Geometry: final body of the model. Coordinates: model frame, mm. A direction names the side the tool comes from. Round coordinates to 2 decimals unless told otherwise and drop trailing zeros. Loops run counter-clockwise (first coordinate to the right, second up) from the corner with the lowest first, then second, coordinate; pieces in that order, holes last. Notation, with made-up numbers: (43, 11.5) - (49, 11.5) arc R21 ccw to (49, 31.5) - close; hole circle Ø7 at (65, 3). An arc over 180 degrees is marked (long way). Answer as CSV lines item,"result".
Autodesk Inventor part; units mm, degrees
ref_plane "YZ Plane" through (0, 0, 0) normal (1, 0, 0) x (0, 1, 0)
ref_plane "XZ Plane" through (0, 0, 0) normal (0, 1, 0) x (-1, 0, 0)
ref_plane "XY Plane" through (0, 0, 0) normal (0, 0, 1) x (1, 0, 0)
sketch "Sketch1" plane through (0, 0, 0) normal (0, 0, 1) x (1, 0, 0)
  circle A0 centre (0, 0) radius 25.4
  dimension "d0" = 50.8
extrude "Extrusion1" add sketch "Sketch1" along normal blind 11.43
sketch "Sketch2" plane through (0, 0, 11.43) normal (0, 0, 1) x (1, 0, 0)
  line L0 (0, 0) -> (-6.35, 0)
  line L1 (0, 0) -> (6.35, 0)
  line L2 (-6.35, 0) -> (-6.35, 6.35)
  line L3 (-6.35, 6.35) -> (-12.7, 6.35)
  line L4 (-12.7, 6.35) -> (-12.7, -6.35)
  line L5 (-12.7, -6.35) -> (-6.35, -6.35)
  line L6 (-6.35, -6.35) -> (-6.35, 0)
  line L7 (6.35, 0) -> (6.35, 6.35)
  line L8 (6.35, 6.35) -> (12.7, 6.35)
  line L9 (12.7, 6.35) -> (12.7, -6.35)
  line L10 (12.7, -6.35) -> (6.35, -6.35)
  line L11 (6.35, -6.35) -> (6.35, 0)
  dimension "d3" = 6.35
  dimension "d4" = 6.35
  dimension "d5" = 6.35
  dimension "d6" = 6.35
  dimension "d7" = 12.7
  dimension "d8" = 6.35
  dimension "d9" = 6.35
  dimension "d10" = 12.7
extrude "Extrusion2" add sketch "Sketch2" along normal blind 22.86
sketch "Sketch3" plane through (0, 0, 34.29) normal (0, 0, 1) x (1, 0, 0)
  line L0 (-12.7, 6.35) -> (-12.7, -6.35)
  line L1 (-12.7, -6.35) -> (-12.7, -8.89)
  line L2 (-12.7, -8.89) -> (-15.24, -8.89)
  line L3 (-15.24, -8.89) -> (15.24, -8.89)
  line L4 (15.24, -8.89) -> (15.24, 8.89)
  line L5 (15.24, 8.89) -> (-15.24, 8.89)
  line L6 (-15.24, 8.89) -> (-15.24, -8.89)
  point P0 (0, 0)
  dimension "d13" = 2.54
  dimension "d14" = 2.54
  dimension "d15" = 30.48
  dimension "d16" = 17.78
extrude "Extrusion3" add sketch "Sketch3" along normal blind 25.4
sketch "Sketch4" plane through (-15.24, -8.89, 34.29) normal (-1, 0, 0) x (0, 0, 1)
  line L0 (0, 17.78) -> (25.4, 17.78)
  line L1 (0, 17.78) -> (0, 12.7)
  line L2 (0, 0) -> (0, 17.78)
  line L3 (0, 12.7) -> (15.24, 12.7)
  line L4 (15.24, 12.7) -> (15.24, 5.08)
  line L5 (15.24, 5.08) -> (21.59, 5.08)
  line L6 (21.59, 5.08) -> (21.59, 12.7)
  line L7 (21.59, 12.7) -> (15.24, 12.7)
  point P0 (-34.29, 8.89)
  dimension "d19" = 5.08
  dimension "d20" = 15.24
  dimension "d21" = 7.62
  dimension "d22" = 6.35
  dimension "d23" = 7.62
extrude "Extrusion4" add sketch "Sketch4" along normal blind 10.16
sketch "Sketch5" plane through (15.24, -8.89, 34.29) normal (1, 0, 0) x (0, 0, -1)
  line L0 (0, 0) -> (0, 5.08)
  line L1 (0, 17.78) -> (0, 0)
  line L2 (0, 5.08) -> (-15.24, 5.08)
  line L3 (-15.24, 5.08) -> (-21.59, 5.08)
  line L4 (-21.59, 5.08) -> (-21.59, 12.7)
  line L5 (-21.59, 12.7) -> (-15.24, 12.7)
  line L6 (-15.24, 12.7) -> (-15.24, 5.08)
  point P0 (34.29, 8.89)
  dimension "d26" = 5.08
  dimension "d27" = 15.24
  dimension "d28" = 6.35
  dimension "d29" = 7.62
extrude "Extrusion5" add sketch "Sketch5" along normal blind 10.16
sketch "Sketch6" plane through (0, 0, 59.69) normal (0, 0, 1) x (1, 0, 0)
  line L0 (-15.24, -8.89) -> (15.24, -8.89)
  line L1 (15.24, -8.89) -> (4.445, -8.89)
  line L2 (-15.24, 8.89) -> (-15.24, -8.89)
  line L3 (-15.24, -8.89) -> (-4.445, -8.89)
  line L4 (-4.445, -8.89) -> (-4.445, -3.81)
  line L5 (15.24, 8.89) -> (-15.24, 8.89)
  line L6 (-4.445, -3.81) -> (4.445, -3.81)
  line L7 (4.445, -3.81) -> (4.445, 3.81)
  line L8 (4.445, 3.81) -> (-4.445, 3.81)
  line L9 (-4.445, 3.81) -> (-4.445, -3.81)
  point P0 (0, 0)
  dimension "d32" = 10.795
  dimension "d33" = 10.795
  dimension "d34" = 5.08
  dimension "d35" = 7.62
extrude "Extrusion6" add sketch "Sketch6" along normal blind 6.35
sketch "Sketch7" plane through (0, 0, 66.04) normal (0, 0, 1) x (1, 0, 0)
  line L0 (4.445, 3.81) -> (4.445, -3.81)
  line L1 (4.445, 3.81) -> (8.255, 3.81)
  line L2 (8.255, 3.81) -> (8.255, 6.35)
  line L3 (12.7, 6.35) -> (6.35, 6.35)
  line L4 (-12.7, -6.35) -> (-6.35, -6.35)
  line L5 (8.255, 6.35) -> (-8.255, 6.35)
  line L6 (-8.255, 6.35) -> (-8.255, -6.35)
  line L7 (-8.255, -6.35) -> (8.255, -6.35)
  line L8 (8.255, -6.35) -> (8.255, 6.35)
  point P0 (0, 0)
  dimension "d38" = 3.81
  dimension "d39" = 16.51
extrude "Extrusion7" add sketch "Sketch7" along normal blind 15.24
sketch "Sketch8" plane through (0, 0, 81.28) normal (0, 0, 1) x (1, 0, 0)
  line L0 (-8.255, 6.35) -> (-8.255, -6.35)
  line L1 (-8.255, -6.35) -> (-8.255, -7.62)
  line L2 (-8.255, -7.62) -> (-9.525, -7.62)
  line L3 (-9.525, -7.62) -> (9.525, -7.62)
  line L4 (9.525, -7.62) -> (9.525, 7.62)
  line L5 (9.525, 7.62) -> (-9.525, 7.62)
  line L6 (-9.525, 7.62) -> (-9.525, -7.62)
  point P0 (0, 0)
  dimension "d42" = 1.27
  dimension "d43" = 1.27
  dimension "d44" = 15.24
extrude "Extrusion8" add sketch "Sketch8" along normal blind 12.7
sketch "Sketch9" plane through (-9.525, 7.62, 81.28) normal (0, 1, 0) x (1, 0, 0)
  line L0 (19.05, 0) -> (0, 0)
  line L1 (19.05, 0) -> (19.05, -12.7)
  line L2 (19.05, -12.7) -> (9.525, -12.7)
  line L3 (19.05, -12.7) -> (0, -12.7)
  line L4 (9.525, -12.7) -> (19.05, 0)
  line L5 (9.525, -12.7) -> (0, -12.7)
  line L6 (0, 0) -> (0, -12.7)
  line L7 (0, 0) -> (0, -12.7)
  line L8 (9.525, -12.7) -> (0, 0)
  point P0 (9.525, 81.28)
sketch "Sketch10" plane through (-9.525, -7.62, 81.28) normal (-1, 0, 0) x (0, 0, 1)
  line L0 (12.7, 0) -> (12.7, 15.24)
  line L1 (12.7, 15.24) -> (12.7, 7.62)
  line L2 (0, 0) -> (0, 15.24)
  line L3 (12.7, 7.62) -> (0, 15.24)
  line L4 (0, 15.24) -> (12.7, 15.24)
  line L5 (0, 0) -> (12.7, 0)
  line L6 (12.7, 0) -> (12.7, 7.62)
  line L7 (12.7, 7.62) -> (0, 0)
  line L8 (12.7, 0) -> (0, 0)
  point P0 (-81.28, 7.62)
  dimension "d47" = 7.62
extrude "Extrusion9" cut sketch "Sketch9" against normal blind 15.24 contours L1 L2 L4 | L8 L3 L6
extrude "Extrusion10" cut sketch "Sketch10" against normal blind 20.32 contours L5 L7 L0 | L3 L4 L0
properties part number "Vasile5-6Bridge.stl"
(1) Section A-A (x = -20). Output: boundary loops of the cut face in (y, z), and give its area (3 significant figures).
Findings below:
outline,"(-15.66, 0) - (15.66, 0) - (15.66, 11.43) - (-15.66, 11.43) - close; (-3.81, 49.53) - (3.81, 49.53) - (3.81, 55.88) - (-3.81, 55.88) - close"
area,"406 mm2"
(2) Pin query (flat end, axial travel): P1, Ø6.5, axis at y = 1.5, z = 18.5, coming from the +X side; P2, Ø5, axis at x = 14, y = -2.5, coming from the +Z side; P3, Ø3, axis at x = 22, z = 51, coming from the -Y side; P4, Ø3, axis at x = -10.5, y = -16.5, coming from the -Z side. Return the tip coordinate at first contact, or that it passes through.
Findings below:
P1,"x = 12.7"
P2,"z = 59.69"
P3,"y = -3.81"
P4,"z = 0"
(3) Section B-B (z = 57.5). Output: boundary loops of the cut face in (x, y).
Findings below:
outline,"(-15.24, -8.89) - (15.24, -8.89) - (15.24, 8.89) - (-15.24, 8.89) - close"
(4) Section C-C (x = 3). Output: boundary loops of the cut face in (y, z), and give its area (3 significant figures).
Findings below:
outline,"(-25.22, 0) - (25.22, 0) - (25.22, 11.43) - (-25.22, 11.43) - close; (-8.89, 34.29) - (8.89, 34.29) - (8.89, 59.69) - (3.81, 59.69) - (3.81, 66.04) - (6.35, 66.04) - (6.35, 81.28) - (7.62, 81.28) - (2.4, 89.98) - (-2.4, 89.98) - (-7.62, 81.28) - (-6.35, 81.28) - (-6.35, 66.04) - (-3.81, 66.04) - (-3.81, 59.69) - (-8.89, 59.69) - close"
area,"1,360 mm2"
(5) Access query for faces 4 (the face through (0, 6.35, 74)), 5 (the face through (8.255, 0, 74)), 6 (the face through (-10, -6.35, 23)), 7 (the face through (0, 4, 59.69)), 8 (the face through (-6.35, 0, 23)). Directions: +Z, -Z, +X, -X, +Y, -Y. A direction counts if a zero-diameter tool reaches every point of the face in a straight line with its end or side. Return the directions, or none.
Findings below:
face 4,"+X, -X, +Y"
face 5,"+X, +Y, -Y"
face 6,"+X, -X, -Y"
face 7,"none"
face 8,"+Y, -Y"
(6) Section D-D (z = 78). Output: boundary loops of the cut face in (x, y) (3 decimals), and give its area (3 significant figures).
Findings below:
outline,"(-8.255, -6.35) - (8.255, -6.35) - (8.255, 6.35) - (-8.255, 6.35) - close"
area,"210 mm2"
(7) Draft query along Z for faces 1 (the face through (-0.13, 4.6, 86.31)), 2 (the face through (9, 6.35, 23)), 3 (the face through (-25.4, 0, 53)). Return one class per face: pulls with the +Z half, pulls with the -Z half, needs draft (parallel to the pull), parting line crosses it, or undercut.
Findings below:
face 1,"pulls with the +Z half"
face 2,"undercut"
face 3,"needs draft"
(8) Material intervals for line 1 along X through (y, z) = (5.5, 30.5); line 2 along Z through (x, y) = (2, -7.5); line 3 along Z through (x, y) = (0.5, -5), sorted ascending.
Findings below:
line 1,"-12.7 to -6.35, 6.35 to 12.7"
line 2,"0 to 11.43, 34.29 to 59.69, 81.28 to 81.48"
line 3,"0 to 11.43, 34.29 to 59.69, 66.04 to 85.65"
